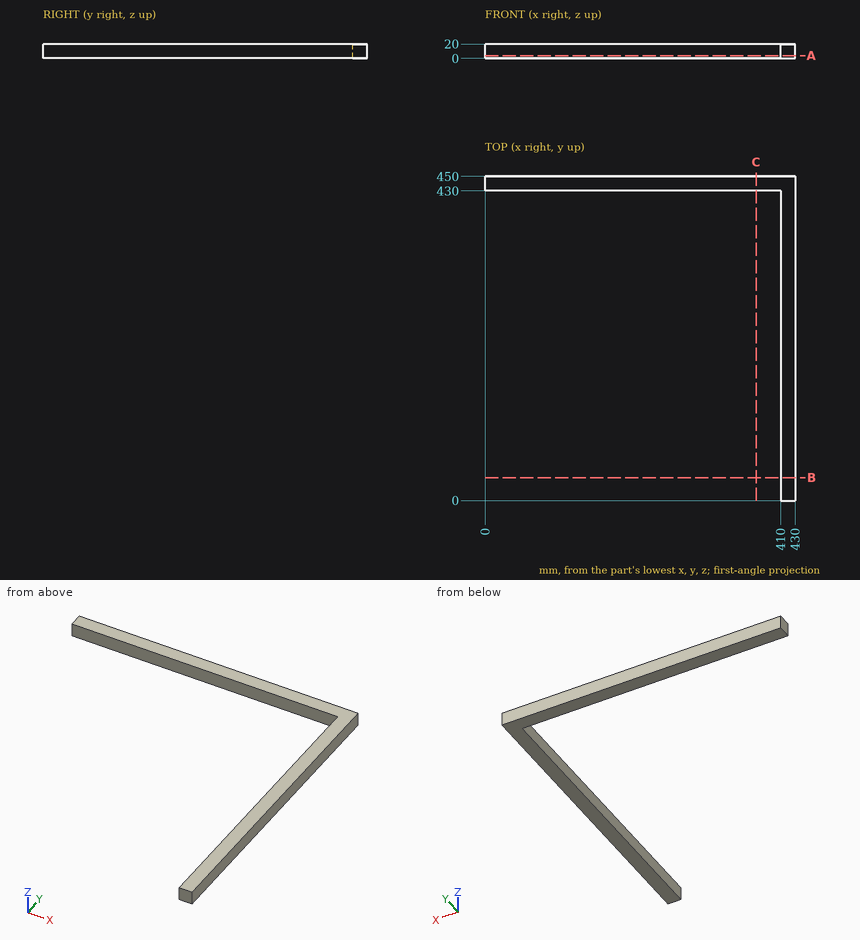
Source: three-view drawing plus pictorial views. Frame: mm from the lowest corner of the part. Coordinates: 2 decimals unless noted, no trailing zeros. Write each loop counter-clockwise with the first axis right and the second up, starting at its lowest first coordinate (ties: lowest second). Pieces come first, ordered by that corner, then holes. Notation, with made-up numbers: (-13.5, 20) - (28.5, 20) arc R18 ccw to (28.5, 34) - close; hole circle Ø8 at (-2, 1.25). An arc over 180 degrees is marked (long way). Answer as a JSON object with one key per item and string values.
Q1. Section query A-A, the plane z = 4. Output: boundary loops of the cut face in (x, y), plus the area to 3 significant figures.
Ans:
{"outline": "(0, 430) - (410, 430) - (410, 0) - (430, 0) - (430, 450) - (0, 450) - close", "area": "17,200 mm2"}
Q2. Material intervals for line 1 (Y direction, x = 231, z = 10.5); line 2 (X direction, y = 319, z = 17.25), sorted ascending. Write a range as [from, to].
Ans:
{"line 1": "y = [430, 450]", "line 2": "x = [410, 430]"}
Q3. Section query B-B, the plane y = 32. Output: boundary loops of the cut face in (x, z).
Ans:
{"outline": "(410, 0) - (430, 0) - (430, 20) - (410, 20) - close"}
Q4. First-contact query: pin 1 Ø1 at (x, z) = (69, 6.5) entering from -Y. Flat tip, straight axial feed; report the tip coordinate or a pass-through.
Ans:
{"pin 1": "stops at y = 430"}
Q5. Section query C-C, the plane x = 376. Output: boundary loops of the cut face in (y, z).
Ans:
{"outline": "(430, 0) - (450, 0) - (450, 20) - (430, 20) - close"}
